Part model, mm, in its own coordinate system. Face numbers are marked on the shaded views. A direction names the side the tool comes from. Round coordinates to 2 decimals unless told otherwise and drop trailing zeros. Write each loop counter-clockwise with the first axis right and the second up, starting at its lowest first coordinate (ties: lowest second). Pieces come first, ordered by that corner, then holes.
1) Saw through at C-C on y = 22.5. Write the cut outline in (x, z), and give its area (3 significant figures).
2) Drill centre lines: L1, parallel to Y at x = -37.5, z = -14.85; L2, parallel to X at y = 14, z = -1; L3, parallel to X at y = 10, z = -15. Where is each one in solid material? Low to high.
3) Saw through at B-B on z = 0. Write the cut outline in (x, y), and give its area (3 significant figures).
4) Pull direction X, two halves, no side cores. Call the marked faces 1, 2 and 3: +X half, -X half, draft (parallel to the pull), parting line (faces both ways), or undercut.
5) Flat gauge pins, fed straight in: pin 1 (5 mm diameter, centred on y = 25, z = 3, fed in from +X); pin 2 (5 mm diameter, centred on x = -38, z = 0, fed in from -Y); pin 3 (9 mm diameter, centred on x = 37.5, y = 28.5, fed in from +Z). Where does each tip first touch, or does it go through?
6) Saw through at A-A on x = -30. Write the cut outline in (y, z).
7) Which spindle directions (+Z, -Z, +X, -X, +Y, -Y) get a long thin tool onto all of the face, cutting with end or side? Do the marked faces 4, 5 and 6. Say none if no direction does.
8) Saw through at D-D on x = 38. Write the cut outline in (y, z), and give its area (3 significant figures).
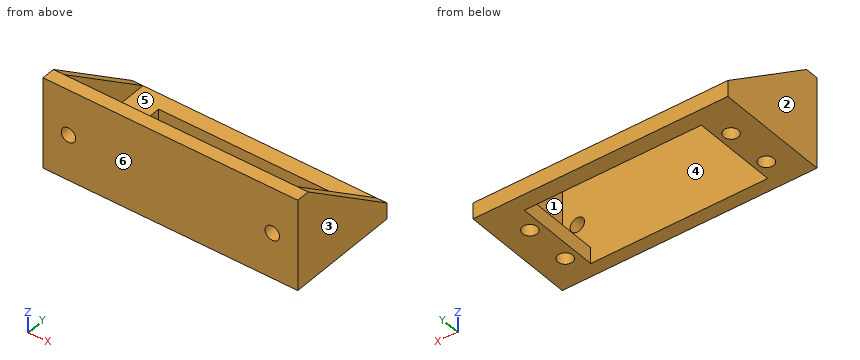
```python
from build123d import *

# Parameters (mm, degrees)
SKETCH1_W           = 95
SKETCH1_H           = 34
BOSS_EXTRUDE1_DEPTH = 5
SKETCH2_W           = 14.5
SKETCH2_H           = 6
BOSS_EXTRUDE2_DEPTH = 38
SKETCH3_W           = 95
SKETCH3_H           = 6
BOSS_EXTRUDE3_DEPTH = 6
SKETCH4_R           = 2.75
CUT_EXTRUDE1_DEPTH  = 6
SKETCH6_R           = 2.7
CUT_EXTRUDE2_DEPTH  = 6
BOSS_EXTRUDE4_DEPTH = 4


with BuildPart() as part:
    # Sketch1 → Boss-Extrude1 (new body)
    with BuildSketch(Plane(origin=(0, 0, 0), x_dir=(1, 0, 0), z_dir=(0, 1, 0))):
        Rectangle(SKETCH1_W, SKETCH1_H)
    extrude(amount=BOSS_EXTRUDE1_DEPTH)

    # Sketch2 → Boss-Extrude2 (add)
    with BuildSketch(Plane(origin=(0, 5, 0), x_dir=(1, 0, 0), z_dir=(0, 1, 0))):
        with Locations((-40.25, 14)):
            Rectangle(SKETCH2_W, SKETCH2_H)
        with Locations((40.25, 14)):
            Rectangle(SKETCH2_W, SKETCH2_H)
    extrude(amount=BOSS_EXTRUDE2_DEPTH)

    # Sketch3 → Boss-Extrude3 (add)
    with BuildSketch(Plane(origin=(0, 43, 0), x_dir=(1, 0, 0), z_dir=(0, 1, 0))):
        with Locations((0, 14)):
            Rectangle(SKETCH3_W, SKETCH3_H)
    extrude(amount=-BOSS_EXTRUDE3_DEPTH)

    # Sketch4 → Cut-Extrude1 (cut)
    with BuildSketch(Plane(origin=(0, 0, -17), x_dir=(-1, 0, 0), z_dir=(0, 0, -1))):
        with Locations((37.5, 11.5)):
            Circle(SKETCH4_R)
        with Locations((37.5, 28.5)):
            Circle(SKETCH4_R)
        with Locations(Location((-37.5, 28.5, 0), (0, 0, 180))):
            Circle(SKETCH4_R)
        with Locations(Location((-37.5, 11.5, 0), (0, 0, 180))):
            Circle(SKETCH4_R)
    extrude(amount=-CUT_EXTRUDE1_DEPTH, mode=Mode.SUBTRACT)

    # Sketch6 → Cut-Extrude2 (cut)
    with BuildSketch(Plane(origin=(0, 5, 0), x_dir=(1, 0, 0), z_dir=(0, 1, 0))):
        with Locations(Location((-38, 0, 0), (0, 0, 270))):
            Circle(SKETCH6_R)
        with Locations(Location((38, 0, 0), (0, 0, 270))):
            Circle(SKETCH6_R)
    extrude(amount=-CUT_EXTRUDE2_DEPTH, mode=Mode.SUBTRACT)

    # Sketch7 → Boss-Extrude4 (add)
    with BuildSketch(Plane.ZY.offset(47.5)):
        Polygon((17, 5), (-11, 43), (-11, 5), align=None)
    boss_extrude4 = extrude(amount=-BOSS_EXTRUDE4_DEPTH)

    # Mirror1: Boss-Extrude4 across plane
    add(boss_extrude4.mirror(Plane(origin=(0, 0, 0), x_dir=(0, 0, 1), z_dir=(1, 0, 0))))


solid = part.part
```
Completed:
1. outline: (-47.5, -17) - (-33, -17) - (-33, -11) - (-43.5, -11) - (-43.5, 4.11) - (-47.5, 4.11) - close; (33, -17) - (47.5, -17) - (47.5, 4.11) - (43.5, 4.11) - (43.5, -11) - (33, -11) - close
1. area: 295 mm2
2. L1: y = 0 to 8.75, 14.25 to 25.75, 31.25 to 43
2. L2: x = -47.5 to -43.5, 43.5 to 47.5
2. L3: x = -47.5 to -39.8, -35.2 to -33, 33 to 35.2, 39.8 to 47.5
3. outline: (-47.5, 0) - (-40.7, 0) - (-40.7, 5) - (-43.5, 5) - (-43.5, 28.07) - (-47.5, 28.07) - close; (-35.3, 0) - (35.3, 0) - (35.3, 5) - (-35.3, 5) - close; (40.7, 0) - (47.5, 0) - (47.5, 28.07) - (43.5, 28.07) - (43.5, 5) - (40.7, 5) - close
3. area: 606 mm2
4. face 1: undercut
4. face 2: -X half
4. face 3: +X half
5. pin 1: stops at x = 47.5
5. pin 2: passes through
5. pin 3: stops at z = -11
6. outline: (0, -17) - (5, -17) - (5, 17) - (0, 17) - close; (37, -17) - (43, -17) - (43, -11) - (37, -11) - close
7. face 4: +Z
7. face 5: +Z, +Y
7. face 6: +Z, -Z, +X, -X, -Y
8. outline: (0, -17) - (8.8, -17) - (8.8, -11) - (5, -11) - (5, -2.7) - (0, -2.7) - close; (0, 2.7) - (5, 2.7) - (5, 17) - (0, 17) - close; (14.2, -17) - (25.8, -17) - (25.8, -11) - (14.2, -11) - close; (31.2, -17) - (43, -17) - (43, -11) - (31.2, -11) - close
8. area: 306 mm2
